CAD build for the part. Positions are in the model's coordinates, mm. Round coordinates to 2 decimals unless told otherwise and drop trailing zeros. Write each loop counter-clockwise with the first axis right and the second up, starting at its lowest first coordinate (ties: lowest second). Pieces come first, ordered by that corner, then holes. Notation, with made-up numbers: (26, -23) - (52, -23) arc R20 cw to (52, -6) - close; hole circle Ø3 at (88.25, 4.25). An arc over 180 degrees is marked (long way). Put each result on its own line as item: value. Start each with the question number.
Item 1: Pin check, flat tips, straight feed: pin 1 Ø2 at (y, z) = (-15.5, 13.5) entering from -X; pin 2 Ø6 at (y, z) = (5, 10.5) entering from +X; pin 3 Ø6 at (x, z) = (1.5, 6.5) entering from -Y; pin 4 Ø4 at (x, y) = (0, 0) entering from +Z. Stop position of each tip, or through.
Item 2: Cut at D-D (z = 6.5). Give the cut face in (x, y).
Item 3: Cut at C-C (z = 13.5). Give the cut face in (x, y).
Item 4: Cut at A-A (x = 0). Give the cut face in (y, z).
Item 5: Drill centre lines: line 1 (Z direction, x = 23, y = -12); line 2 (Y direction, x = 0, z = 6.5); line 3 (Y direction, x = 1, z = 10). Where is each one in solid material? Low to high. Write a range as from..to.
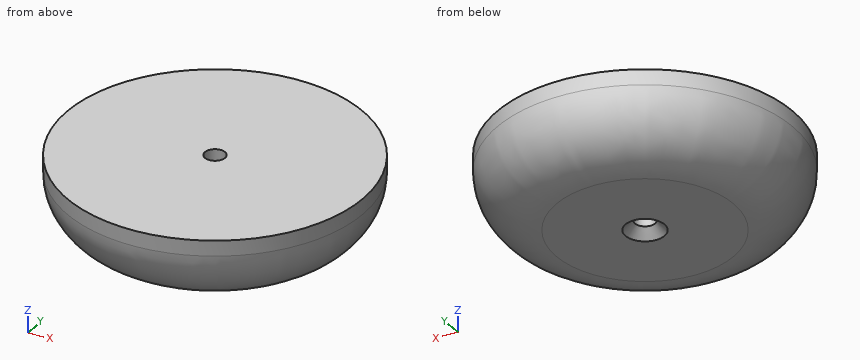
```python
from build123d import *

# Parameters (mm, degrees)
F0_R     = 31.75
F1_DEPTH = 16.002
F2_R     = 12.7
F3_R     = 2.159
F4_DEPTH = 16.003
F5_SIZE  = 2.032


with BuildPart() as f1:
    # F0 (on Top) → F1 (new body)
    with BuildSketch(Plane.XY):
        Circle(F0_R)
    extrude(amount=F1_DEPTH)

    # F2
    f2_edges = [f1.edges().sort_by_distance(p)[0] for p in [
        (-31.75, 0, 0),
    ]]
    fillet(f2_edges, radius=F2_R)

    # F3 (on face) → F4 (cut, through all)
    with BuildSketch(Plane.XY.offset(16.002)):
        Circle(F3_R)
    extrude(amount=-F4_DEPTH, mode=Mode.SUBTRACT)

    # F5
    f5_edges = [f1.edges().sort_by_distance(p)[0] for p in [
        (-2.159, 0, 0),
    ]]
    chamfer(f5_edges, length=F5_SIZE)


solid = f1.part
```
Output values:
1. pin 1: x = -28.25
1. pin 2: x = 31.64
1. pin 3: y = -31.31
1. pin 4: through
2. outline: circle Ø60.27 at (0, 0); hole circle Ø4.32 at (0, 0)
3. outline: circle Ø63.5 at (0, 0); hole circle Ø4.32 at (0, 0)
4. outline: (-31.75, 12.7) arc R12.7 ccw to (-19.05, 0) - (-4.19, 0) - (-2.16, 2.03) - (-2.16, 16) - (-31.75, 16) - close; (2.16, 2.03) - (4.19, 0) - (19.05, 0) arc R12.7 ccw to (31.75, 12.7) - (31.75, 16) - (2.16, 16) - close
5. line 1: 2.03..16
5. line 2: -30.13..-2.16, 2.16..30.13
5. line 3: -31.44..-1.91, 1.91..31.44
